Work out the finished part from the listing and answer in its coordinate system (mm). Give positions to 0.01 mm unless a question says otherwise; leave off trailing zeros. Loops run counter-clockwise (first coordinate to the right, second up) from the corner with the lowest first, then second, coordinate; pieces in that order, holes last. Notation, with made-up numbers: M 10.25,68.25 L 41.25,68.25 A6 cw 41.25,75.25 Z; hole C 58.5,-14.75 d10. An arc over 180 degrees is marked long. Use a Markdown table: item, result.
```python
from build123d import *

# Parameters (mm, degrees)
SKETCH1_R           = 2.5
BOSS_EXTRUDE1_DEPTH = 1.95
CUT_EXTRUDE1_DEPTH  = 1.06


with BuildPart() as part:
    # Sketch1 → Boss-Extrude1 (new, symmetric)
    with BuildSketch(Plane.XY):
        with BuildLine():
            Line((34.5, -4.3), (-34.5, -4.3))
            ThreePointArc((-34.5, -4.3), (-38.8, 0), (-34.5, 4.3))
            Line((-34.5, 4.3), (34.5, 4.3))
            ThreePointArc((34.5, 4.3), (38.8, 0), (34.5, -4.3))
        make_face()
        with Locations((-34.5, 0)):
            Circle(SKETCH1_R, mode=Mode.SUBTRACT)
        with Locations((34.5, 0)):
            Circle(SKETCH1_R, mode=Mode.SUBTRACT)
    extrude(amount=BOSS_EXTRUDE1_DEPTH, both=True)

    # Sketch2 → Cut-Extrude1 (cut)
    with BuildSketch(Plane.XY.offset(1.95)):
        with BuildLine():
            ThreePointArc((30.747667392, -2.1), (30.2, 0), (30.747667392, 2.1))
            Line((30.747667392, 2.1), (-30.747667392, 2.1))
            ThreePointArc((-30.747667392, 2.1), (-30.33916894, 1.08511976), (-30.2, 0))
            ThreePointArc((-30.2, 0), (-30.33916894, -1.08511976), (-30.747667392, -2.1))
            Line((-30.747667392, -2.1), (30.747667392, -2.1))
        make_face()
    cut_extrude1 = extrude(amount=-CUT_EXTRUDE1_DEPTH, mode=Mode.SUBTRACT)

    # Mirror1: Cut-Extrude1 across plane
    add(cut_extrude1.mirror(Plane.XY), mode=Mode.SUBTRACT)


solid = part.part
```
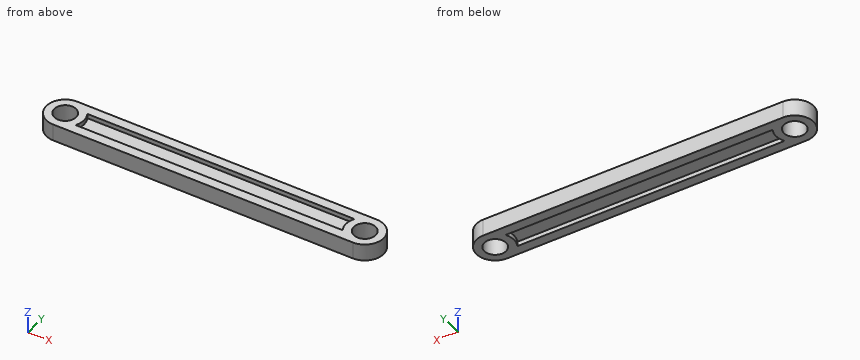
(1) A cutting plane is placed at B-B (y = 3.25). Write down the section's boundary in (x, z).
Entries:
| item | result |
|---|---|
| outline | M -37.32,-1.95 L 37.32,-1.95 L 37.32,1.95 L -37.32,1.95 Z |
(2) Consider probe 1 along Y at (x, z) = (24, 0.95); probe 2 along Y at (x, z) = (34.5, -0.85); probe 3 along X at (y, z) = (2, -0.35). Determine where each line is inside the solid, lowest interval first. Write a range as [from, to].
Entries:
| item | result |
|---|---|
| probe 1 | y = [-4.3, -2.1], [2.1, 4.3] |
| probe 2 | y = [-4.3, -2.5], [2.5, 4.3] |
| probe 3 | x = [-38.31, -36], [-33, 33], [36, 38.31] |
(3) A cutting plane is placed at A-A (x = 3.5). Write down the section's boundary in (y, z), and give its area (3 significant figures).
Entries:
| item | result |
|---|---|
| outline | M -4.3,-1.95 L -2.1,-1.95 L -2.1,-0.89 L 2.1,-0.89 L 2.1,-1.95 L 4.3,-1.95 L 4.3,1.95 L 2.1,1.95 L 2.1,0.89 L -2.1,0.89 L -2.1,1.95 L -4.3,1.95 Z |
| area | 24.6 mm² |
(4) Given P1, Ø1, axis at y = -2, z = 1, coming from the +X side; P2, Ø4.5, axis at x = 34.5, y = 0, coming from the +Z side, each flat-ended and moving along its own axis, determine where each tip first touches the part or whether it passes through.
Entries:
| item | result |
|---|---|
| P1 | stops at x = 38.53 |
| P2 | passes through |
